Design review of the part shown in the three views and the two pictorial views. Dimensions are in mm from the part's minimum x, y and z. A direction names the side the tool comes from. Coordinates: 2 decimals unless noted, no trailing zeros. Loops run counter-clockwise (first coordinate to the right, second up) from the corner with the lowest first, then second, coordinate; pieces in that order, holes last.
Q1. Wall thickness on probe 1 along X at (y, z) = (0.15, 12.5); probe 2 along X at (y, z) = (2.75, 12.5); probe 3 along Y at (x, z) = (7, 13): over which ranges is each line inside the solid? List them lowest first.
Q2. Add section D-D on z = 23. Give the boundary of the cut face in (x, y).
Q3. Add section B-B on z = 12.5. Give the boundary of the cut face in (x, y), and give its area (3 significant figures).
Q4. Machinability: for the marked faces 1, 2 and 3, which of the approach directions +Z, -Z, +X, -X, +Y, -Y give a long, thin tool a straight path to every point of the face, cutting with its end or side? Answer none if there is none.
Q5. Add section C-C on y = 5. Give the boundary of the cut face in (x, z).
Q6. For P1, Ø1, axis at y = 3.5, z = 17.5, coming from the -X side; P2, Ø2, axis at y = 1.5, z = 20.5, coming from the -X side; P3, Ø2, axis at x = 3, y = 3, coming from the -Z side; P4, Ø6.5, axis at x = 12.5, z = 12.5, coming from the -Y side, all flat-tipped, find the tip position at first contact; note any pin that passes through.
Q7. Add section A-A on x = 12.5. Give the boundary of the cut face in (y, z), and give its area (3 significant figures).
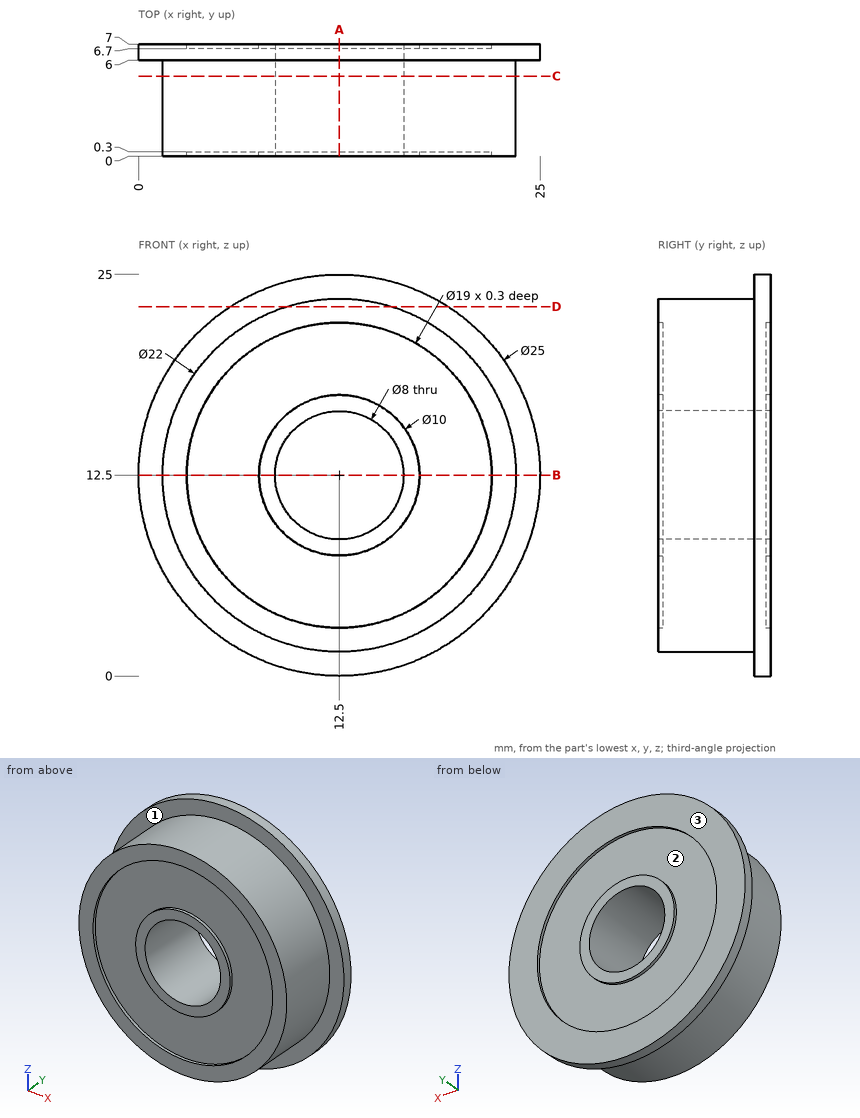
Entries:
1. probe 1: x = 1.5 to 3, 7.5 to 8.5, 16.5 to 17.5, 22 to 23.5
1. probe 2: x = 1.5 to 8.5, 16.5 to 23.5
1. probe 3: y = 0.3 to 6.7
2. outline: (5.72, 6) - (9.22, 6) - (9.22, 0) - (15.78, 0) - (15.78, 6) - (19.28, 6) - (19.28, 7) - (5.72, 7) - close
3. outline: (0, 6) - (1.5, 6) - (1.5, 0) - (3, 0) - (3, 0.3) - (7.5, 0.3) - (7.5, 0) - (8.5, 0) - (8.5, 7) - (7.5, 7) - (7.5, 6.7) - (3, 6.7) - (3, 7) - (0, 7) - close; (16.5, 0) - (17.5, 0) - (17.5, 0.3) - (22, 0.3) - (22, 0) - (23.5, 0) - (23.5, 6) - (25, 6) - (25, 7) - (22, 7) - (22, 6.7) - (17.5, 6.7) - (17.5, 7) - (16.5, 7) - close
3. area: 95.6 mm2
4. face 1: -Y
4. face 2: +Y
4. face 3: +Z, -Z, +X, -X, +Y
5. outline: circle Ø22 at (12.5, 12.5); hole circle Ø8 at (12.5, 12.5)
6. P1: stops at x = 2.46
6. P2: stops at x = 4.01
6. P3: stops at z = 5.52
6. P4: passes through
7. outline: (0, 1.5) - (6, 1.5) - (6, 0) - (7, 0) - (7, 3) - (6.7, 3) - (6.7, 7.5) - (7, 7.5) - (7, 8.5) - (0, 8.5) - (0, 7.5) - (0.3, 7.5) - (0.3, 3) - (0, 3) - close; (0, 16.5) - (7, 16.5) - (7, 17.5) - (6.7, 17.5) - (6.7, 22) - (7, 22) - (7, 25) - (6, 25) - (6, 23.5) - (0, 23.5) - (0, 22) - (0.3, 22) - (0.3, 17.5) - (0, 17.5) - close
7. area: 95.6 mm2
